Build history of the part. All positions in model axes, mm. A direction names the side the tool comes from. Give positions to 0.01 mm unless a question says otherwise; leave off trailing zeros. Write each loop counter-clockwise with the first axis right and the second up, starting at its lowest first coordinate (ties: lowest second). Pieces come first, ordered by that corner, then holes. Notation, with made-up numbers: (43, -17) -> (52, -17) arc R18 cw to (52, 4) -> close; hole circle Ø3 at (82, 25). An arc over 180 degrees is marked (long way). Write item = value, one per line. Start each with the question number.
Q1. Tool access for faces 1 (the face through (13, 0, -29.115)), 2 (the face through (13, -2.095, -4)), 3 (the face through (25.4, -49, -19)), 4 (the face through (13, -51.845, 22)): list every direction of +Z, -Z, +X, -X, +Y, -Y with a clear straight run to the whole face (end or side of a thin tool).
Q2. Wall check: line 1 (Z direction, x = 13.75, y = -39.5); line 2 (Z direction, x = 12, y = -1); line 3 (Y direction, x = 16, z = -97). Give the ranges that are in metal, low to high.
Q3. Saw through at A-A, the plane z = 15. List the corners of the cut face in (x, y).
Q4. Saw through at B-B, the plane x = 22.25. List the corners of the cut face in (y, z).
Q5. Mould opens along Y. For faces 5 (the face through (13, -25, 20.885)), 6 (the face through (13, 1.655, -3)), 7 (the face through (3.61, -50.44, -106.66)) say: pulls with the +Y half, pulls with the -Y half, needs draft (parallel to the pull), parting line crosses it, or undercut.
Q6. Drop flat-ended pins along their axis: P1, Ø7.5, axis at x = 13, y = -30.5, coming from the -Z side; P2, Ø7.5, axis at x = 15.5, z = -3, coming from the -Y side; P3, Ø1, axis at x = 7.5, z = -30.5, coming from the +Y side; P4, Ø12, axis at y = -38.5, z = -41, coming from the -X side. Give the stop position or say it passes through.
Q7. Saw through at C-C, the plane y = -4. List the corners of the cut face in (x, z), then the cut area to 3 significant figures.
Q8. Saw through at D-D, the plane z = -53. List the corners of the cut face in (x, y).
from build123d import *

# Parameters (mm, degrees)
F0_W     = 3.75
F0_H     = 50
F1_DEPTH = 25.4
F2_R     = 1.5
F3_DEPTH = 3.75
F4_R     = 12.6501077242


with BuildPart() as f1:
    # F0 (on Right) → F1 (new body)
    with BuildSketch(Plane.YZ):
        Polygon((-51.8451631069, 20.965634957), (-48.095487799, 20.8846080303), (-2.095487799, 20.8846080303), (1.654512201, 20.8846080303), (1.654512201, 23.4246080303), (-51.8451631069, 23.4246080303), align=None)
        Polygon((-48.6218297482, -110.4640364647), (-48.095487799, 20.8846080303), (-51.8451631069, 20.965634957), (-52.3718297482, -110.4640364647), align=None)
        with Locations((-0.220487799, -4.1153919697)):
            Rectangle(F0_W, F0_H)
    extrude(amount=F1_DEPTH)

    # F2 (on face) → F3 (cut)
    with BuildSketch(Plane(origin=(0, -51.9283430119, 0.2080879127), x_dir=(1, 0, 0), z_dir=(0, -0.9999919712, 0.0040071805))):
        with Locations((12.722876047, -99.3401251781)):
            Circle(F2_R)
    extrude(amount=-F3_DEPTH, mode=Mode.SUBTRACT)

    # F4
    f4_edges = [f1.edges().sort_by_distance(p)[0] for p in [
        (25.4, -50.49683, -110.464036),
        (0, -50.49683, -110.464036),
    ]]
    fillet(f4_edges, radius=F4_R)


solid = f1.part
Report:
q1.face_1 = -Z, +X, -X, +Y
q1.face_2 = -Z, +X, -X
q1.face_3 = +Z, -Z, +X, +Y, -Y
q1.face_4 = +Z, +X, -X, -Y
q2.line_1 = 20.88 to 23.42
q2.line_2 = -29.12 to 23.42
q2.line_3 = -52.32 to -48.57
q3.outline = (0, -51.87) -> (25.4, -51.87) -> (25.4, -48.12) -> (0, -48.12) -> close; (0, -2.1) -> (25.4, -2.1) -> (25.4, 1.65) -> (0, 1.65) -> close
q4.outline = (-52.35, -106.17) -> (-48.6, -106.17) -> (-48.1, 20.88) -> (-2.1, 20.88) -> (-2.1, -29.12) -> (1.65, -29.12) -> (1.65, 23.42) -> (-51.85, 23.42) -> (-51.85, 20.97) -> close
q5.face_5 = undercut
q5.face_6 = pulls with the +Y half
q5.face_7 = needs draft
q6.P1 = 20.88
q6.P2 = -51.96
q6.P3 = -48.3
q6.P4 = through
q7.outline = (0, 20.88) -> (25.4, 20.88) -> (25.4, 23.42) -> (0, 23.42) -> close
q7.area = 64.5 mm2
q8.outline = (0, -52.14) -> (25.4, -52.14) -> (25.4, -48.39) -> (0, -48.39) -> close
